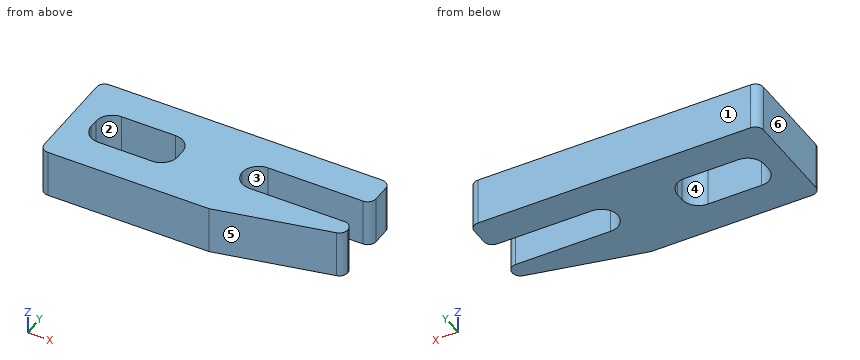
from build123d import *

# Parameters (mm, degrees)
F0_W     = 35
F0_H     = 13.2
F1_DEPTH = 5.76
F2_W     = 10.5
F2_H     = 5
F2_W_2   = 15
F2_H_2   = 4
F3_DEPTH = 25
F4_R     = 1.99999
F5_R     = 1


# Not quite as in the source:
# - a fillet or chamfer is up to 0.001 mm smaller than in the source, because OpenCascade refuses the exact size


with BuildPart() as f1:
    # F0 (on Top) → F1 (new body)
    with BuildSketch(Plane.XY):
        with Locations((-7.6907900348, 3.6986840781)):
            Rectangle(F0_W, F0_H)
    extrude(amount=F1_DEPTH)

    # F2 (on face) → F3 (cut)
    with BuildSketch(Plane.XY.offset(5.76)):
        Polygon((-4.6907900348, -2.9013159219), (9.8092099652, -2.9013159219), (9.8092099652, 0.2986840781), align=None)
        with Locations((-17.1407900348, 3.6986840781)):
            Rectangle(F2_W, F2_H)
        with Locations((2.8092099652, 4.1986840781)):
            Rectangle(F2_W_2, F2_H_2)
    extrude(amount=-F3_DEPTH, mode=Mode.SUBTRACT)

    # F4 (radius 2 in the source; OpenCascade refuses exactly that, so slightly less here)
    f4_edges = [f1.edges().sort_by_distance(p)[0] for p in [
        (-22.39079, 6.198684, 2.88),
        (-11.89079, 6.198684, 2.88),
        (-11.89079, 1.198684, 2.88),
        (-22.39079, 1.198684, 2.88),
        (-4.69079, 2.198684, 2.88),
        (-4.69079, 6.198684, 2.88),
    ]]
    fillet(f4_edges, radius=F4_R)

    # F5
    f5_edges = [f1.edges().sort_by_distance(p)[0] for p in [
        (9.80921, 10.298684, 2.88),
        (9.80921, 6.198684, 2.88),
        (9.80921, 2.198684, 2.88),
        (9.80921, 0.298684, 2.88),
        (-25.19079, -2.901316, 2.88),
        (-25.19079, 10.298684, 2.88),
    ]]
    fillet(f5_edges, radius=F5_R)


solid = f1.part
Input: part model. Units: mm. Frame: model coordinates. Face numbers are marked on the shaded views. A direction names the side the tool comes from. Give positions to 0.01 mm unless a question says otherwise; leave off trailing zeros. Loops run counter-clockwise (first coordinate to the right, second up) from the corner with the lowest first, then second, coordinate; pieces in that order, holes last. Notation, with made-up numbers: M 36,-8.75 L 57,-8.75 A25 cw 57,6.25 Z; hole C -3,-32 d7. An arc over 180 degrees is marked long. Use CSV: the item, a comma, the result in double quotes.
(1) Pin query (flat end, axial travel): P1, Ø1.7, axis at x = 1, z = 2.5, coming from the -Y side; P2, Ø0.5, axis at y = 3.5, z = 2, coming from the +X side. Return the tip coordinate at first contact, or that it passes through.
Outcome:
P1,"stops at y = -1.83"
P2,"stops at x = -4.45"
(2) Section A-A, the plane x = -15.5. Return loops of the section in (y, z), plus the area to 3 significant figures.
Outcome:
outline,"M -2.9,0 L 1.2,0 L 1.2,5.76 L -2.9,5.76 Z; M 6.2,0 L 10.3,0 L 10.3,5.76 L 6.2,5.76 Z"
area,"47.2 mm²"
(3) Set-up query: the marked faces 1, 2 and 3. Return all of +Z, -Z, +X, -X, +Y, -Y with unobstructed straight access to the full face (end or side cutting, diameter ignored); none if empty.
Outcome:
face 1,"+Z, -Z, +X, -X, +Y"
face 2,"+Z, -Z"
face 3,"+Z, -Z, +X"
(4) Pull-direction query (Y, two-part tool) for the marked faces 4, 5 and 6; classes: pulls with the +Y half, pulls with the -Y half, needs draft (parallel to the pull), parting line crosses it, or undercut.
Outcome:
face 4,"undercut"
face 5,"pulls with the -Y half"
face 6,"needs draft"
(5) Section C-C, the plane y = 3.75. Return loops of the section in (x, z), plus the area to 3 significant figures.
Outcome:
outline,"M -25.19,0 L -22.39,0 L -22.39,5.76 L -25.19,5.76 Z; M -11.89,0 L -4.64,0 L -4.64,5.76 L -11.89,5.76 Z"
area,"57.9 mm²"
(6) Material intervals for L1, parallel to Y at x = -16, z = 4.65; L2, parallel to X at y = 2, z = 4.65; L3, parallel to Y at x = -1.5, z = 2.8, sorted ascending. Write a range as [from, to].
Outcome:
L1,"y = [-2.9, 1.2], [6.2, 10.3]"
L2,"x = [-25.19, -21.99], [-12.29, 9.41]"
L3,"y = [-2.2, 2.2], [6.2, 10.3]"
